from build123d import *

# Parameters (mm, degrees)
FURO_ROSCADO_DE_M61_D           = 5
FURO_ROSCADO_DE_M61_CSINK_D     = 6.05
FURO_ROSCADO_DE_M61_CSINK_ANGLE = 90
CHANFRO1_SIZE                   = 0.2
CHANFRO3_SIZE                   = 3
CHANFRO3_SIZE2                  = 0.803847577
CORTE_EXTRUS_O1_REACH           = 31.306
CORTE_EXTRUS_O1_END_RADIUS      = 6.25
ESBO_O7_R                       = 1.35


with BuildPart() as part:
    # Esboço1 → Revolução1 (revolve)
    with BuildSketch(Plane(origin=(0, 0, 0), x_dir=(1, 0, 0), z_dir=(0, 1, 0)), mode=Mode.PRIVATE) as revolu_o1_sk:
        Polygon((-0.058940995, 6.25), (27.941059005, 6.25), (27.941059005, 0), (19.941059005, 0), (19.941059005, 5), (-0.058940995, 5), align=None)
    revolve(revolu_o1_sk.sketch.rotate(Axis((0, 0, 0), (1, 0, 0)), 180), axis=Axis((0, 0, 0), (1, 0, 0)))

    # Furo roscado de M61 (through all)
    with Locations(Plane(origin=(27.941059005, 0, 0), x_dir=(0, 0, -1), z_dir=(1, 0, 0))):
        with Locations((0, 0)):
            CounterSinkHole(FURO_ROSCADO_DE_M61_D / 2, FURO_ROSCADO_DE_M61_CSINK_D / 2, counter_sink_angle=FURO_ROSCADO_DE_M61_CSINK_ANGLE)

    # Chanfro1
    chanfro1_edges = [part.edges().sort_by_distance(p)[0] for p in [
        (27.941059005, 0, -6.25),
    ]]
    chamfer(chanfro1_edges, length=CHANFRO1_SIZE)

    # Chanfro3
    chanfro3_edges = [part.edges().sort_by_distance(p)[0] for p in [
        (-0.058940995, 0, -6.25),
    ]]
    chanfro3_side = [part.faces().sort_by_distance(p)[0] for p in [
        (13.841059005, 0, -6.25),
    ]]
    chamfer(chanfro3_edges, length=CHANFRO3_SIZE, length2=CHANFRO3_SIZE2, reference=chanfro3_side[0])

    # Corte-extrusão1: up to this cylinder (the profile starts inside it)
    corte_extrus_o1_end = Plane(origin=(23.941059, 0, 0), z_dir=(-1, 0, 0)) * Cylinder(CORTE_EXTRUS_O1_END_RADIUS, 76.112, mode=Mode.PRIVATE)
    # Esboço7 → Corte-extrusão1 (cut, up to the surface)
    with BuildSketch(Plane(origin=(0, 0, 0), x_dir=(1, 0, 0), z_dir=(0, 1, 0)), mode=Mode.PRIVATE) as corte_extrus_o1_sk1:
        with Locations(Location((23.941059005, 0, 0), (0, 0, 270))):
            Circle(ESBO_O7_R)
    corte_extrus_o1_tool1 = extrude(corte_extrus_o1_sk1.sketch, amount=-CORTE_EXTRUS_O1_REACH, mode=Mode.PRIVATE) & corte_extrus_o1_end
    add(corte_extrus_o1_tool1.solids().sort_by_distance((23.941059, 0, 0))[0], mode=Mode.SUBTRACT)


solid = part.part
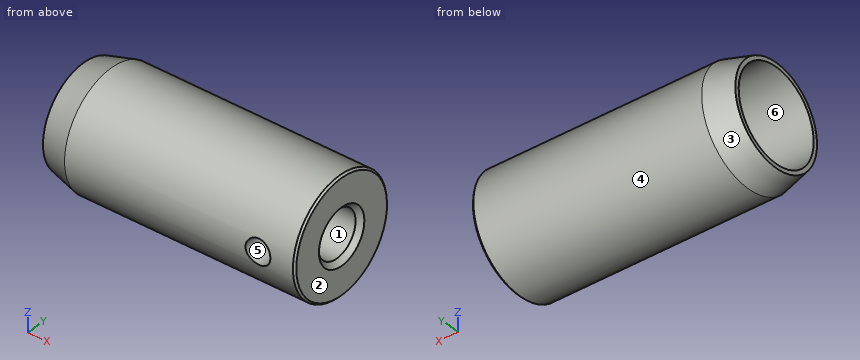
Verification items for the finished model (mm, model axes). Face numbers are marked on the shaded views. A direction names the side the tool comes from. Give positions to 0.01 mm unless a question says otherwise; leave off trailing zeros. Loops run counter-clockwise (first coordinate to the right, second up) from the corner with the lowest first, then second, coordinate; pieces in that order, holes last.
1) Set-up check for the marked faces 4, 5 and 6: record each of +Z, -Z, +X, -X, +Y, -Y from which the full face is reachable in a straight line by a thin tool's end or side.
2) Thickness scan on line 1 along Y through (x, z) = (22.5, 0); line 2 along X through (y, z) = (-4.45, 0); line 3 along X through (y, z) = (-5.1, 0). Record the ranges inside material, lowest first.
3) Sectioned sample at C-C, the plane x = 14. Enter the section's corners in (y, z).
4) Sectioned sample at A-A, the plane y = 0. Enter the section's corners in (x, z) (3 decimals).
5) Sectioned sample at B-B, the plane z = 0. Enter the section's corners in (x, y) (3 decimals).
6) Depth check by flat-ended pin: pin 1 Ø3 at (x, z) = (25, -0.5) entering from +Y; pin 2 Ø3 at (y, z) = (-1, -2.5) entering from -X; pin 3 Ø5 at (x, y) = (9, -4) entering from +Z; pin 4 Ø4 at (x, y) = (15, 5) entering from +Z. Enter the tip coordinate at first touch or a pass-through.
7) Draft check along Y on the marked faces 1, 2 and 3. Enter one of: pulls with the +Y half, pulls with the -Y half, needs draft (parallel to the pull), parting line crosses it, or undercut.
Answers:
1. face 4: +X, -X
1. face 5: -Y
1. face 6: -X
2. line 1: y = -6.25 to -2.5, 2.5 to 6.25
2. line 2: x = 19.94 to 22.59, 25.29 to 27.94
2. line 3: x = -0.06 to 22.59, 25.29 to 27.94
3. outline: circle Ø12.5 at (0, 0); hole circle Ø10 at (0, 0)
4. outline: (-0.059, -5.446) - (2.941, -6.25) - (27.741, -6.25) - (27.941, -6.05) - (27.941, -3.025) - (27.416, -2.5) - (19.941, -2.5) - (19.941, -5) - (-0.059, -5) - close; (-0.059, 5) - (19.941, 5) - (19.941, 2.5) - (27.416, 2.5) - (27.941, 3.025) - (27.941, 6.05) - (27.741, 6.25) - (2.941, 6.25) - (-0.059, 5.446) - close
5. outline: (-0.059, -5.446) - (2.941, -6.25) - (22.591, -6.25) - (22.591, -2.5) - (19.941, -2.5) - (19.941, -5) - (-0.059, -5) - close; (-0.059, 5) - (19.941, 5) - (19.941, 2.5) - (27.416, 2.5) - (27.941, 3.025) - (27.941, 6.05) - (27.741, 6.25) - (2.941, 6.25) - (-0.059, 5.446) - close; (25.291, -6.25) - (27.741, -6.25) - (27.941, -6.05) - (27.941, -3.025) - (27.416, -2.5) - (25.291, -2.5) - close
6. pin 1: stops at y = 6.25
6. pin 2: stops at x = 19.94
6. pin 3: stops at z = 6.07
6. pin 4: stops at z = 5.48
7. face 1: undercut
7. face 2: needs draft
7. face 3: parting line crosses it
